Input: part model. Units: mm. Frame: model coordinates. Round coordinates to 2 decimals unless told otherwise and drop trailing zeros. Write each loop counter-clockwise with the first axis right and the second up, starting at its lowest first coordinate (ties: lowest second). Pieces come first, ordered by that corner, then holes. Notation, with made-up numbers: (-12, 43.25) -> (36, 43.25) arc R22 cw to (36, 77.25) -> close; hole circle Ø9 at (83.25, 8). An arc over 180 degrees is marked (long way). Write item = value, one per line.
```python
from build123d import *

# Parameters (mm, degrees)
SKETCH1_W                                    = 114.3
SKETCH1_H                                    = 111.252
BOSS_EXTRUDE1_DEPTH                          = 1.27
CSK_FOR_M2_5_COUNTERSUNK_FLAT_HEAD_S_2_COUNT = 2
CSK_FOR_M2_5_COUNTERSUNK_FLAT_HEAD_S_2_PITCH = 104.140077439
CSK_FOR_M2_5_COUNTERSUNK_FLAT_HEAD_S_3_COUNT = 2
CSK_FOR_M2_5_COUNTERSUNK_FLAT_HEAD_S_3_PITCH = 145.225430146
CSK_FOR_M2_5_COUNTERSUNK_FLAT_HEAD_S_4_COUNT = 2
CSK_FOR_M2_5_COUNTERSUNK_FLAT_HEAD_S_4_PITCH = 101.219
FILLET1_R                                    = 1.27
SKETCH9_W                                    = 30.48
SKETCH9_H                                    = 90.932
CUT_EXTRUDE5_DEPTH                           = 5.08


with BuildPart() as part:
    # Sketch1 → Boss-Extrude1 (new body)
    with BuildSketch(Plane(origin=(0, 0, 0), x_dir=(1, 0, 0), z_dir=(0, 1, 0))):
        with Locations((-13.076419672, -24.671311475)):
            Rectangle(SKETCH1_W, SKETCH1_H)
    extrude(amount=BOSS_EXTRUDE1_DEPTH)

    # Sketch3 → CSK for M2.5 Countersunk Flat Head Screw1 (revolve, cut)
    with BuildSketch(Plane(origin=(-65.146419672, 1.27, -26.001688525), x_dir=(0, 0, 1), z_dir=(1, 0, 0))):
        Polygon((0, 0), (0, 1.27), (1.45, 1.27), (1.45, 1.3), (2.75, 0), align=None)
    csk_for_m2_5_countersunk_flat_head_screw = revolve(axis=Axis((-65.146419672, 7.62, -26.001688525), (0, -1, 0)), mode=Mode.SUBTRACT)

    # CSK for M2.5 Countersunk Flat Head S 2: CSK for M2.5 Countersunk Flat Head Screw1 ×2
    with Locations(*[Vector(0.9999992563958324, 0, 0.0012195112882876242) * (i * CSK_FOR_M2_5_COUNTERSUNK_FLAT_HEAD_S_2_PITCH) for i in range(1, CSK_FOR_M2_5_COUNTERSUNK_FLAT_HEAD_S_2_COUNT)]):
        add(csk_for_m2_5_countersunk_flat_head_screw, mode=Mode.SUBTRACT)

    # CSK for M2.5 Countersunk Flat Head S 3: CSK for M2.5 Countersunk Flat Head Screw1 ×2
    with Locations(*[Vector(0.7170920402544414, 0, 0.6969784830277923) * (i * CSK_FOR_M2_5_COUNTERSUNK_FLAT_HEAD_S_3_PITCH) for i in range(1, CSK_FOR_M2_5_COUNTERSUNK_FLAT_HEAD_S_3_COUNT)]):
        add(csk_for_m2_5_countersunk_flat_head_screw, mode=Mode.SUBTRACT)

    # CSK for M2.5 Countersunk Flat Head S 4: CSK for M2.5 Countersunk Flat Head Screw1 ×2
    with Locations(*[(0, 0, i * CSK_FOR_M2_5_COUNTERSUNK_FLAT_HEAD_S_4_PITCH) for i in range(1, CSK_FOR_M2_5_COUNTERSUNK_FLAT_HEAD_S_4_COUNT)]):
        add(csk_for_m2_5_countersunk_flat_head_screw, mode=Mode.SUBTRACT)

    # Fillet1
    fillet1_edges = [part.edges().sort_by_distance(p)[0] for p in [
        (-70.226419672, 0.635, -30.954688525),
        (44.073580328, 0.635, -30.954688525),
        (44.073580328, 0.635, 80.297311475),
        (-70.226419672, 0.635, 80.297311475),
    ]]
    fillet(fillet1_edges, radius=FILLET1_R)

    # Sketch9 → Cut-Extrude5 (cut)
    with BuildSketch(Plane(origin=(0, 1.27, 0), x_dir=(1, 0, 0), z_dir=(0, 1, 0))):
        with Locations((28.833580328, -24.671311475)):
            Rectangle(SKETCH9_W, SKETCH9_H)
        with Locations((-54.986419672, -24.671311475)):
            Rectangle(SKETCH9_W, SKETCH9_H)
    extrude(amount=-CUT_EXTRUDE5_DEPTH, mode=Mode.SUBTRACT)


solid = part.part
```
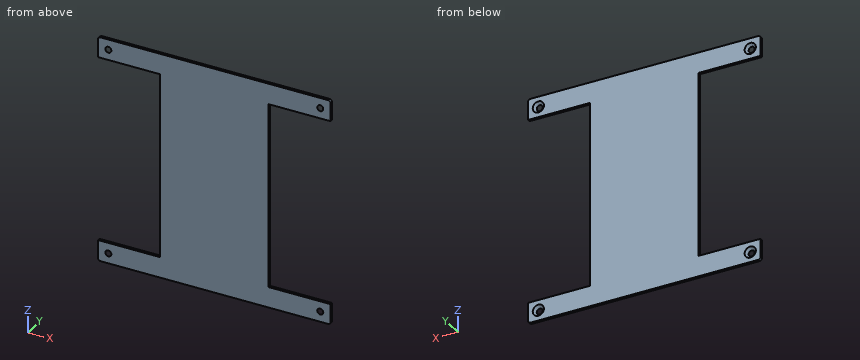
1) First-contact query: P1, Ø0.6, axis at y = 0.5, z = 25, coming from the -X side. Flat tip, straight axial feed; report the tip coordinate or a pass-through.
Solutions:
P1 = -39.75
2) Cut plane C-C (z = -9.5). Return the cut outline in (x, y).
Solutions:
outline = (-39.75, 0) -> (13.59, 0) -> (13.59, 1.27) -> (-39.75, 1.27) -> close
3) Cut plane A-A (x = 23). Return the cut outline in (y, z), and give its area (3 significant figures).
Solutions:
outline = (0, -30.95) -> (1.27, -30.95) -> (1.27, -20.79) -> (0, -20.79) -> close; (0, 70.14) -> (1.27, 70.14) -> (1.27, 80.3) -> (0, 80.3) -> close
area = 25.8 mm^2
4) Line query: L1, parallel to Z at x = 36, y = 0.95; L2, parallel to X at y = 0.65, z = 5.5; L3, parallel to X at y = 0.25, z = 74. Output: solid intervals per line, ascending. Write a range as from..to.
Solutions:
L1 = -30.95..-20.79, 70.14..80.3
L2 = -39.75..13.59
L3 = -70.23..-66.38, -63.92..37.76, 40.22..44.07
5) Cut plane B-B (y = 0.5). Return the cut outline in (x, z).
Solutions:
outline = (-70.23, -29.68) arc R1.27 ccw to (-68.96, -30.95) -> (42.8, -30.95) arc R1.27 ccw to (44.07, -29.68) -> (44.07, -20.79) -> (13.59, -20.79) -> (13.59, 70.14) -> (44.07, 70.14) -> (44.07, 79.03) arc R1.27 ccw to (42.8, 80.3) -> (-68.96, 80.3) arc R1.27 ccw to (-70.23, 79.03) -> (-70.23, 70.14) -> (-39.75, 70.14) -> (-39.75, -20.79) -> (-70.23, -20.79) -> close; hole circle Ø3.96 at (-65.15, -26); hole circle Ø3.96 at (-65.15, 75.22); hole circle Ø3.96 at (38.99, -25.87); hole circle Ø3.96 at (38.99, 75.22)
